Geometry check sheet. Reference: the model listing, model coordinates, mm. Round coordinates to 2 decimals unless told otherwise and drop trailing zeros. Order: outer loops, then holes, each group sorted by start corner. A loop starts at its lowest first (then second) coordinate and runs counter-clockwise, first axis right, second up. Notation, with made-up numbers: (71.5, 60) - (127.5, 60) arc R13 ccw to (127.5, 82) - close; hole circle Ø10 at (35.25, -15.5). An arc over 180 degrees is marked (long way). Return JSON: item names as keys, results as strings. Group by question number.
Q1. Material ranges on line 1 along Z through (x, y) = (-22, 10.5); line 2 along Z through (x, y) = (-3, 3.75); line 3 along X through (y, z) = (5.5, 1.5), recorded low to high.
Q2. Sectioned sample at A-A, the plane x = 18.5. Record the cut outline in (y, z).
Q3. Draft check along Z on faces 1 (the cylindrical face through (11.985, 6.902, -0.66)), 2 (the flat face through (25, 7, 0)), 3 (the flat face through (-3, 7, -25)). Enter one of: pulls with the +Z half, pulls with the -Z half, needs draft (parallel to the pull), parting line crosses it, or undercut.
Q4. Sectioned sample at D-D, the plane y = 12. Record the cut outline in (x, z), then the cut area to 3 significant figures.
Q5. Gauge pin test, flat end, axial feed: pin 1 Ø12 at (x, z) = (-6.5, 8) entering from +Y. Record the tip position at first contact, or that the pin passes through.
Q6. Sectioned sample at C-C, the plane z = 16. Record the cut outline in (x, y).
Q7. Sectioned sample at B-B, the plane x = -22. Record the cut outline in (y, z).
Autodesk Inventor part; units mm, degrees
ref_plane "YZ Plane" through (0, 0, 0) normal (1, 0, 0) x (0, 1, 0)
ref_plane "XZ Plane" through (0, 0, 0) normal (0, 1, 0) x (-1, 0, 0)
ref_plane "XY Plane" through (0, 0, 0) normal (0, 0, 1) x (1, 0, 0)
sketch "Szkic1" plane through (0, 0, 0) normal (0, 1, 0) x (-1, 0, 0)
  circle A0 centre (3, 0) radius 15
  line L0 (32, -51.5) -> (19.7697, -51.5)
  arc A1 (19.7697, -48.5) -> (19.7697, -51.5) centre (15, -50) ccw
  line L1 (19.7697, -48.5) -> (32, -48.5)
  line L2 (32, 48.5) -> (32, -48.5)
  line L3 (32, 48.5) -> (19.7697, 48.5)
  arc A2 (19.7697, 51.5) -> (19.7697, 48.5) centre (15, 50) ccw
  line L4 (19.7697, 51.5) -> (32, 51.5)
  line L5 (32, 60) -> (32, 51.5)
  line L6 (32, 60) -> (-25, 60)
  line L7 (-25, 60) -> (-25, -60)
  line L8 (-25, -60) -> (32, -60)
  line L9 (32, -51.5) -> (32, -60)
  line L10 (-25, 0) -> (-25, -25)
  line L11 (-25, -25) -> (32, -25)
  line L12 (-25, 0) -> (-25, 25)
  line L13 (-25, 25) -> (32, 25)
  point P0 (0, 0)
  point P1 (0, 0)
  dimension "d0" = 25
  dimension "d1" = 25
extrude "Wyciągnięcie proste1" add sketch "Szkic1" along normal blind 14 contours L7 L13 L2 L11
sketch "Szkic2" plane through (0, 14, 0) normal (0, 1, 0) x (1, 0, 0)
  circle A0 centre (-3, 0) radius 15
  line L0 (-32, 25) -> (-32, -25)
  line L1 (25, -25) -> (25, 25)
  line L2 (12, 0) -> (15, 0)
  line L3 (-18, 0) -> (-22, 0)
  line L4 (-22, 0) -> (-22, 16)
  line L5 (-22, 0) -> (-22, -16)
  circle A1 centre (-22, 16) radius 2.5
  circle A2 centre (-22, -16) radius 2.5
  line L6 (12, 0) -> (18.5, 0)
  circle A3 centre (18.5, 0) radius 2.5
  point P0 (0, 0)
  dimension "d11" = 10
  dimension "d12" = 5
  dimension "d13" = 5
  dimension "d18" = 6.5
  dimension "d19" = 5
extrude "Wyciągnięcie proste2" cut sketch "Szkic2" against normal up to next contours A2 | A1 | A3
properties part number "Uchwyt górnego łożyska osi Z"
Reply:
{
 "1": {"line 1": "-25 to -18.5, -13.5 to 13.5, 18.5 to 25", "line 2": "-25 to -15, 15 to 25", "line 3": "-32 to -17.92, 11.92 to 16.5, 20.5 to 25"},
 "2": {"outline": "(0, -25) - (14, -25) - (14, -2.5) - (0, -2.5) - close; (0, 2.5) - (14, 2.5) - (14, 25) - (0, 25) - close"},
 "3": {"face 1": "undercut", "face 2": "needs draft", "face 3": "pulls with the -Z half"},
 "4": {"outline": "(-32, -25) - (25, -25) - (25, 25) - (-32, 25) - close; hole circle Ø5 at (-22, -16); hole circle Ø5 at (-22, 16); hole circle Ø30 at (-3, 0); hole circle Ø5 at (18.5, 0)", "area": "2,080 mm^2"},
 "5": {"pin 1": "through"},
 "6": {"outline": "(-32, 0) - (-24.5, 0) - (-24.5, 14) - (-32, 14) - close; (-19.5, 0) - (25, 0) - (25, 14) - (-19.5, 14) - close"},
 "7": {"outline": "(0, -25) - (14, -25) - (14, -18.5) - (0, -18.5) - close; (0, -13.5) - (14, -13.5) - (14, 13.5) - (0, 13.5) - close; (0, 18.5) - (14, 18.5) - (14, 25) - (0, 25) - close"}
}
